Verification items for the finished model (mm, model axes). A direction names the side the tool comes from. Round coordinates to 2 decimals unless told otherwise and drop trailing zeros. Order: outer loops, then holes, each group sorted by start corner. A loop starts at its lowest first (then second) coordinate and runs counter-clockwise, first axis right, second up. Notation, with made-up numbers: M -18.75,-25 L 16.25,-25 A12 cw 16.25,-10 Z; hole C -17.75,57 d1. An arc over 180 degrees is marked long. Answer as a JSON object with one key per item and string values. Group by question number.
```python
from build123d import *

# Parameters (mm, degrees)
CROQUIS1_W     = 30
CROQUIS1_H     = 30
EXTRUIR1_DEPTH = 30
CROQUIS5_W     = 30
CROQUIS5_H     = 30
EXTRUIR4_DEPTH = 30
CROQUIS2_W     = 30
CROQUIS2_H     = 30
CROQUIS2_W_2   = 24
CROQUIS2_H_2   = 24
EXTRUIR2_DEPTH = 30
CROQUIS3_W     = 30
CROQUIS3_H     = 30
CROQUIS3_W_2   = 24
CROQUIS3_H_2   = 24
EXTRUIR3_DEPTH = 30
CROQUIS7_W     = 30
CROQUIS7_H     = 30
CROQUIS7_W_2   = 24
CROQUIS7_H_2   = 24
EXTRUIR5_DEPTH = 30
VACIADO1_T     = -5


with BuildPart() as part:
    # Croquis1 → Extruir1 (new body)
    with BuildSketch(Plane(origin=(0, 0, 0), x_dir=(1, 0, 0), z_dir=(0, 1, 0))):
        with Locations((0, 30)):
            Rectangle(CROQUIS1_W, CROQUIS1_H)
        Rectangle(CROQUIS1_W, CROQUIS1_H)
        with Locations((30, 0)):
            Rectangle(CROQUIS1_W, CROQUIS1_H)
    extrude(amount=EXTRUIR1_DEPTH)

    # Croquis5 → Extruir4 (add)
    with BuildSketch(Plane.XZ):
        Rectangle(CROQUIS5_W, CROQUIS5_H)
    extrude(amount=EXTRUIR4_DEPTH)

    # Croquis2 → Extruir2 (cut)
    with BuildSketch(Plane(origin=(45, 0, 0), x_dir=(0, 0, -1), z_dir=(1, 0, 0))):
        with Locations((0, 15)):
            Rectangle(CROQUIS2_W, CROQUIS2_H)
        with Locations((0, 15)):
            Rectangle(CROQUIS2_W_2, CROQUIS2_H_2, mode=Mode.SUBTRACT)
    extrude(amount=-EXTRUIR2_DEPTH, mode=Mode.SUBTRACT)

    # Croquis3 → Extruir3 (cut)
    with BuildSketch(Plane(origin=(0, 0, -45), x_dir=(-1, 0, 0), z_dir=(0, 0, -1))):
        with Locations((0, 15)):
            Rectangle(CROQUIS3_W, CROQUIS3_H)
        with Locations((0, 15)):
            Rectangle(CROQUIS3_W_2, CROQUIS3_H_2, mode=Mode.SUBTRACT)
    extrude(amount=-EXTRUIR3_DEPTH, mode=Mode.SUBTRACT)

    # Croquis7 → Extruir5 (cut)
    with BuildSketch(Plane.XZ.offset(30)):
        Rectangle(CROQUIS7_W, CROQUIS7_H)
        Rectangle(CROQUIS7_W_2, CROQUIS7_H_2, mode=Mode.SUBTRACT)
    extrude(amount=-EXTRUIR5_DEPTH, mode=Mode.SUBTRACT)

    # Vaciado1
    vaciado1_openings = [part.faces().sort_by_distance(p)[0] for p in [
        (45, 15, 0),
        (0, 15, -45),
        (0, -30, 0),
    ]]
    offset(amount=VACIADO1_T, openings=vaciado1_openings, kind=Kind.INTERSECTION)


solid = part.part
```
Q1. Release check for a two-part mould opening along X. For faces 5 (the face through (45, 7, 0)), 6 (the face through (-15, 15, 0)), 7 (the face through (0, 15, 10)) record: released by +X, released by -X, zero draft, split by the parting line, or undercut.
Q2. Cross-section at C-C, the plane x = 11. Record the cut outline in (y, z).
Q3. Tool access check on faces 1 (the face through (12, -15, 0)), 2 (the face through (28, 15, 7)), 3 (the face through (0, -13, -7)), 4 (the face through (7, 15, -28)). Record the directions out of +Z, -Z, +X, -X, +Y, -Y that give a thin tool (end or side, any length) a straight path to the whole face; none if there is none.
Q4. Gauge pin test, flat ends, axial feed: pin 1 Ø4 at (y, z) = (23, -25) entering from -X; pin 2 Ø7 at (y, z) = (16, -22) entering from +X; pin 3 Ø15.5 at (x, y) = (28, 12.5) entering from +Z. Record the tip position at first contact, or that the pin passes through.
Q5. Thickness scan on line 1 (Y direction, x = -5, z = 9.5); line 2 (Y direction, x = 14, z = -6); line 3 (Z direction, x = 25.5, y = 11.5). Record the ranges inside material, lowest first. Write a range as from..to.
Q6. Cross-section at D-D, the plane z = -32. Record the cut outline in (x, y), then the cut area to 3 significant figures.
Q7. Cross-section at B-B, the plane x = 0.5. Record the cut outline in (y, z), then the cut area to 3 significant figures.
Q8. Cross-section at A-A, the plane y = 17.5. Record the cut outline in (x, z), then the cut area to 3 significant figures.
Conclusion:
{
 "1": {"face 5": "released by +X", "face 6": "released by -X", "face 7": "undercut"},
 "2": {"outline": "M -30,-12 L 0,-12 L 0,-15 L 3,-15 L 3,-45 L 27,-45 L 27,-15 L 30,-15 L 30,15 L 0,15 L 0,12 L -30,12 Z; hole M 8,-7 L 22,-7 L 22,7 L 8,7 Z"},
 "3": {"face 1": "+Z, -Z, +X, -Y", "face 2": "+X", "face 3": "-Y", "face 4": "-Z"},
 "4": {"pin 1": "x = -12", "pin 2": "x = 12", "pin 3": "z = 12"},
 "5": {"line 1": "-30..5, 25..30", "line 2": "0..8, 22..30", "line 3": "-12..-7, 7..12"},
 "6": {"outline": "M -12,3 L 12,3 L 12,27 L -12,27 Z; hole M -7,8 L 7,8 L 7,22 L -7,22 Z", "area": "380 mm2"},
 "7": {"outline": "M -30,-12 L 0,-12 L 0,-15 L 3,-15 L 3,-45 L 8,-45 L 8,-10 L 5,-10 L 5,-7 L -30,-7 Z; M -30,7 L 5,7 L 5,10 L 25,10 L 25,-10 L 22,-10 L 22,-45 L 27,-45 L 27,-15 L 30,-15 L 30,15 L 0,15 L 0,12 L -30,12 Z", "area": "960 mm2"},
 "8": {"outline": "M -15,-15 L -12,-15 L -12,-45 L -7,-45 L -7,-10 L -10,-10 L -10,10 L 10,10 L 10,7 L 45,7 L 45,12 L 15,12 L 15,15 L -15,15 Z; M 7,-45 L 12,-45 L 12,-15 L 15,-15 L 15,-12 L 45,-12 L 45,-7 L 10,-7 L 10,-10 L 7,-10 Z", "area": "960 mm2"}
}
